from build123d import *

# Parameters (mm, degrees)
SKETCH_R        = 2.25
PAD_DEPTH       = 23
POCKET_DEPTH    = 19
SKETCH002_R     = 4.05
SKETCH002_R_2   = 2.25
POCKET001_DEPTH = 20.001
SKETCH003_R     = 2.25
POCKET002_DEPTH = 10
SKETCH004_R     = 3.75
POCKET003_DEPTH = 10
SKETCH005_R     = 3.75
POCKET004_DEPTH = 10


with BuildPart() as pocket004:
    # Sketch → Pad (new body)
    with BuildSketch(Plane.XY):
        Polygon((0, -20), (40, -20), (40, 20), (-20, 20), (-20, 0), (0, 0), align=None)
        with Locations((15, 8)):
            Circle(SKETCH_R, mode=Mode.SUBTRACT)
        with Locations((10, -10)):
            Circle(SKETCH_R, mode=Mode.SUBTRACT)
        with Locations((25, -10)):
            Circle(SKETCH_R, mode=Mode.SUBTRACT)
    extrude(amount=PAD_DEPTH)

    # Sketch001 → Pocket (cut)
    with BuildSketch(Plane.XY.offset(23)):
        with BuildLine():
            Line((46, 10), (26, 10))
            ThreePointArc((26, 10), (22.778175, 17.778175), (15, 21))
            Line((15, 21), (0, 21))
            Line((0, 21), (0, -23))
            Line((0, -23), (46, -23))
            Line((46, -23), (46, -12))
            Line((25.538775, -14.46763), (46, -12))
            ThreePointArc((25.538775, -5.53237), (20.5, -10), (25.538775, -14.46763))
            Line((25.538775, -5.53237), (46, -8))
            Line((46, -8), (46, 10))
        make_face()
    extrude(amount=-POCKET_DEPTH, mode=Mode.SUBTRACT)

    # Sketch002 → Pocket001 (cut, through all)
    with BuildSketch(Plane.XZ):
        with Locations((-7, 16)):
            Circle(SKETCH002_R)
        with Locations((-10, 6)):
            Circle(SKETCH002_R_2)
    extrude(amount=-POCKET001_DEPTH, mode=Mode.SUBTRACT)

    # Sketch003 → Pocket002 (cut)
    with BuildSketch(Plane.XY.offset(23)):
        with Locations((35, 15)):
            Circle(SKETCH003_R)
    extrude(amount=-POCKET002_DEPTH, mode=Mode.SUBTRACT)

    # Sketch004 → Pocket003 (cut)
    with BuildSketch(Plane(origin=(0, 20, 0), x_dir=(-1, 0, 0), z_dir=(0, 1, 0))):
        with Locations((10, 6)):
            Circle(SKETCH004_R)
    extrude(amount=-POCKET003_DEPTH, mode=Mode.SUBTRACT)

    # Sketch005 → Pocket004 (cut)
    with BuildSketch(Plane(origin=(0, 0, 0), x_dir=(1, 0, 0), z_dir=(0, 0, -1))):
        with Locations((25, 10)):
            Circle(SKETCH005_R)
    extrude(amount=-POCKET004_DEPTH, mode=Mode.SUBTRACT)


with BuildPart() as part_mirroring:
    # Part__Mirroring: instance of Pocket004
    add(pocket004.part.mirror(Plane(origin=(0, 0, 0), x_dir=(0, -1, 0), z_dir=(1, 0, 0))))


solid = part_mirroring.part
The model under review builds one solid part; all positions refer to its coordinate system, in mm. A direction names the side the tool comes from. Give positions to 0.01 mm unless a question says otherwise; leave off trailing zeros. Write each loop counter-clockwise with the first axis right and the second up, starting at its lowest first coordinate (ties: lowest second). Pieces come first, ordered by that corner, then holes. Notation, with made-up numbers: M -21.5,-30.5 L 14.5,-30.5 A34 ccw 14.5,-0.5 Z; hole C -40,43.5 d2. An arc over 180 degrees is marked long. One line per question, with ' | ' between items. Start each with the question number.
Item 1: Wall thickness on line 1 (Z direction, x = 7, y = 13.75); line 2 (Y direction, x = -25, z = 5.25); line 3 (Z direction, x = 8.5, y = 8.5): over which ranges is each line inside the solid? List them lowest first. Write a range as from..to.
Item 2: We need section A-A on z = 9. Write out the cut boundary in (x, y).
Item 3: For faces 1 (the cylindrical face through (7.878, 9.86, 12.046)), 2 (the cylindrical face through (-36.038, 13.004, 18.07)), 3 (the cylindrical face through (-26.21, -8.103, 16.409)), 4 (the cylindrical face through (7.024, 15.07, 3.718)), 5 (the flat face through (-32.668, -6.392, 13.633)), list the 3-axis set-ups (+Z, -Z, +X, -X, +Y, -Y) from which the entire face can be reached by the end or side of a thin tool; tool diameter is ignored.
Item 4: We need section D-D on z = 21.75. Write out the cut boundary in (x, y).
Item 5: We need section B-B on x = -15. Write out the cut boundary in (y, z).
Item 6: For pin 1 (10 mm diameter, centred on x = 0, z = 10.5, fed in from -Y); pin 2 (1 mm diameter, centred on x = 8, z = 3.5, fed in from +Y); pin 3 (1.5 mm diameter, centred on x = -17, y = 16, fed in from +Z), all flat-tipped, find the tip position at first contact; note any pin that passes through.
Item 7: We need section C-C on y = 8. Write out the cut boundary in (x, z), plus the area to 3 significant figures.
Item 8: Draft analysis for pull direction Y (two halves, no side actions). For faces 6 (the flat face through (12, 10, 4)), 7 (the flat face through (0, 10, 14)), 8 (the cylindrical face through (-8.34, -8.48, 1.97)), state which applies: released by +Y, released by -Y, zero draft, split by the parting line, or undercut.
Results found:
1) line 1: z = 0..3.75, 8.25..11.95, 20.05..23 | line 2: y = -14.5..-13.75, -6.25..-5.5, 14.58..20 | line 3: z = 0..4.32, 7.68..12.24, 19.76..23
2) outline: M -40,-12.72 L -25.54,-14.47 A4.5 ccw long -25.54,-5.53 L -40,-7.28 Z; M -40,10 L -26,10 A11 cw -19.58,20 L -40,20 Z; M 0,0 L 20,0 L 20,20 L 12.25,20 L 12.25,10 L 7.75,10 L 7.75,20 L 0,20 Z; hole C -25,-10 d7.5
3) face 1: +Y, -Y | face 2: +Z | face 3: +Z, -Z | face 4: +Y | face 5: +Z, -X
4) outline: M -40,-12.72 L -25.54,-14.47 A4.5 ccw long -25.54,-5.53 L -40,-7.28 Z; M -40,10 L -26,10 A11 cw -19.58,20 L -40,20 Z; M 0,0 L 20,0 L 20,20 L 0,20 Z; hole C -35,15 d4.5; hole C -25,-10 d4.5
5) outline: M -20,0 L 5.75,0 L 5.75,4 L -20,4 Z; M 10.25,0 L 20,0 L 20,4 L 10.25,4 Z
6) pin 1: stops at y = 0 | pin 2: stops at y = 10 | pin 3: stops at z = 4
7) outline: M -40,0 L -17.25,0 L -17.25,4 L -40,4 Z; M -12.75,0 L 20,0 L 20,23 L 0,23 L 0,4 L -12.75,4 Z; hole C 7,16 d8.1; hole C 10,6 d4.5 | area: 535 mm2
8) face 6: released by +Y | face 7: zero draft | face 8: undercut
